```python
from build123d import *

# Parameters (mm, degrees)
SKETCH_2_R          = 6
EXTRUDE_1_DEPTH     = 20
FILLET_1_R          = 8.5
SKETCH_3_W          = 3
SKETCH_3_H          = 0.5
CUT_EXTRUDE_1_DEPTH = 100
CUT_EXTRUDE_2_DEPTH = 100


with BuildPart() as part:
    # 草图2 → 凸台-拉伸1 (new body)
    with BuildSketch(Plane.XY):
        with BuildLine():
            ThreePointArc((23, 8.5), (37.51040764, 14.51040764), (31.5, 0))
            Line((31.5, 0), (23, 0))
            Line((23, 0), (20, 0))
            Line((20, 0), (0, 0))
            Line((0, 0), (0, 5))
            Line((0, 5), (23, 5))
            Line((23, 5), (23, 8.5))
        make_face()
        with Locations((31.5, 8.5)):
            Circle(SKETCH_2_R, mode=Mode.SUBTRACT)
    extrude(amount=EXTRUDE_1_DEPTH)

    # 圆角1
    fillet_1_edges = [part.edges().sort_by_distance(p)[0] for p in [
        (23, 5, 10),
    ]]
    fillet(fillet_1_edges, radius=FILLET_1_R)

    # 草图3 → 切除-拉伸1 (cut)
    with BuildSketch(Plane.XY.offset(20)):
        with Locations((21.5, 0.25)):
            Rectangle(SKETCH_3_W, SKETCH_3_H)
    extrude(amount=-CUT_EXTRUDE_1_DEPTH, mode=Mode.SUBTRACT)

    # 草图4 → 切除-拉伸2 (cut)
    with BuildSketch(Plane.XY.offset(20)):
        Polygon((23, 0), (23.5, 0), (23, 0.5), align=None)
        Polygon((20, 0), (19.5, 0), (20, 0.5), align=None)
    extrude(amount=-CUT_EXTRUDE_2_DEPTH, mode=Mode.SUBTRACT)


solid = part.part
```
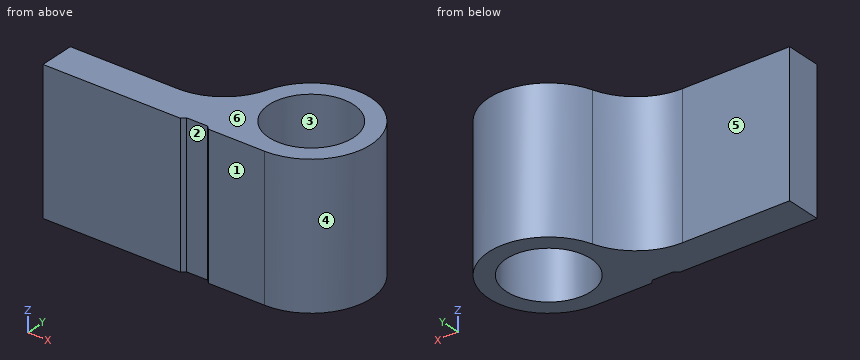
Read the model definition and answer for the solid it produces. Units are mm, in the model's axes. Face numbers are marked on the shaded views. A direction names the side the tool comes from. Round coordinates to 2 decimals unless told otherwise and drop trailing zeros. Loops run counter-clockwise (first coordinate to the right, second up) from the corner with the lowest first, then second, coordinate; pieces in that order, holes last. Notation, with made-up numbers: (-12, 67) -> (18, 67) arc R6 cw to (18, 76) -> close; hole circle Ø10 at (70.25, -23.5). An arc over 180 degrees is marked (long way). One line per item, written item: value.
1) A cutting plane is placed at B-B (y = 12.75). Determine the outline of the cut face in (x, z), and give its area (3 significant figures).
Answer list:
outline: (24.14, 0) -> (27.26, 0) -> (27.26, 20) -> (24.14, 20) -> close; (35.74, 0) -> (38.86, 0) -> (38.86, 20) -> (35.74, 20) -> close
area: 125 mm²
2) A cutting plane is placed at C-C (x = 3.5). Determine the outline of the cut face in (y, z).
Answer list:
outline: (0, 0) -> (5, 0) -> (5, 20) -> (0, 20) -> close
3) The mould has two halves that part along X. Classify the marked faces 1, 2, 3 and 4: pulls with the +X half, pulls with the -X half, needs draft (parallel to the pull), parting line crosses it, or undercut.
Answer list:
face 1: needs draft
face 2: undercut
face 3: undercut
face 4: parting line crosses it
4) A cutting plane is placed at A-A (x = 36). Determine the outline of the cut face in (y, z), and give its area (3 significant figures).
Answer list:
outline: (1.29, 0) -> (4.53, 0) -> (4.53, 20) -> (1.29, 20) -> close; (12.47, 0) -> (15.71, 0) -> (15.71, 20) -> (12.47, 20) -> close
area: 130 mm²
5) Consider L1, parallel to Y at x = 31.5, z = 10.5; L2, parallel to Y at x = 8, z = 16; L3, parallel to X at y = 3, z = 8. Determine where each line is inside the solid, lowest interval first. Write a range as [from, to].
Answer list:
L1: y = [0, 2.5], [14.5, 17]
L2: y = [0, 5]
L3: x = [0, 29.1], [33.9, 37.98]
6) For the marked faces 5 and 6, determine the directions among +Z, -Z, +X, -X, +Y, -Y from which every point of the face is accessible in a straight line to the end or side of a thin tool.
Answer list:
face 5: +Z, -Z, -X, +Y
face 6: +Z, +X, -X, +Y, -Y
7) Flat-ended cylindrical pins translate along their axes: P1, Ø8, axis at y = 15, z = 8, coming from the +X side; P2, Ø2.5, axis at x = 22, z = 5.5, coming from the -Y side; P3, Ø5, axis at x = 30, y = 6.5, coming from the +Z side; P4, Ø1.5, axis at x = 25, z = 8.5, coming from the +Y side. Find the tip coordinate at first contact, or state that the pin passes through.
Answer list:
P1: stops at x = 39.62
P2: stops at y = 0.25
P3: passes through
P4: stops at y = 14.76
